```python
from build123d import *

# Parameters (mm, degrees)
SKETCH1_14_W = 152.4
SKETCH1_14_H = 20


with BuildPart() as part:
    # Sketch1<14> → Revolve9 (revolve)
    with BuildSketch(Plane.YZ, mode=Mode.PRIVATE) as revolve9_sk:
        with Locations((76.2, 4077.73873053)):
            Rectangle(SKETCH1_14_W, SKETCH1_14_H)
    revolve(revolve9_sk.sketch.rotate(Axis((0, 0, 4067.73873053), (0, 0, 1)), 90), axis=Axis((0, 0, 4067.73873053), (0, 0, 1)))

    # Sketch1<18> → Revolve-Thin9 (revolve)
    with BuildSketch(Plane.YZ):
        with BuildLine():
            ThreePointArc((0, 5357.73873053), (6.238377253, 5355.554269491), (9.751256095, 5349.955260381))
            ThreePointArc((9.751256095, 5349.955260381), (115.877016875, 4722.808595757), (151.4, 4087.73873053))
            Line((151.4, 4087.73873053), (150.4, 4087.73873053))
            ThreePointArc((150.4, 4087.73873053), (114.883254929, 4722.697073583), (8.776130485, 5349.733607396))
            ThreePointArc((8.776130485, 5349.733607396), (5.614539527, 5354.772715595), (0, 5356.73873053))
            Line((0, 5356.73873053), (0, 5357.73873053))
        make_face()
    revolve(axis=Axis((0, 0, 2579.7350764), (0, 0, 1)))


solid = part.part
```
Here's how the part is built. I have some questions about the finished solid (model axes, mm). Give positions to 0.01 mm unless a question says otherwise; leave off trailing zeros. Put each result on its own line as item: value. Start each with the question number.
Item 1: Thinking about a two-plate mould opening in X: for faces 1 (the flat face through (-2, -2, 4067.739)), 2 (the flat face through (-2, -2, 4087.739)), 3 (the cylindrical face through (33.037, 148.776, 4077.879)), which applies, +X half, -X half, draft (parallel to the pull), parting line (faces both ways), or undercut?
Item 2: Will these pins go through, and if not, where does the flat tip stop? pin 1 (1 mm diameter, centred on x = 62, z = 4732.5, fed in from -Y); pin 2 (10 mm diameter, centred on y = 80, z = 4627, fed in from -X); pin 3 (8 mm diameter, centred on x = 102, z = 4736.5, fed in from -Y).
Item 3: I need wall thicknesses on L1, parallel to X at y = 20.5, z = 4541.5; L2, parallel to Y at x = 2, z = 4557.5; L3, parallel to Y at x = 58.5, z = 4599.5. Which ranges of each line are inside material? Lowest first, please. Write a range as from..to.
Values:
1. face 1: draft
1. face 2: undercut
1. face 3: parting line
2. pin 1: y = -96.92
2. pin 2: x = -101.06
2. pin 3: y = -58.93
3. L1: -131.71..-130.69, 130.69..131.71
3. L2: -131.98..-130.97, 130.97..131.98
3. L3: -114.25..-113.12, 113.12..114.25
